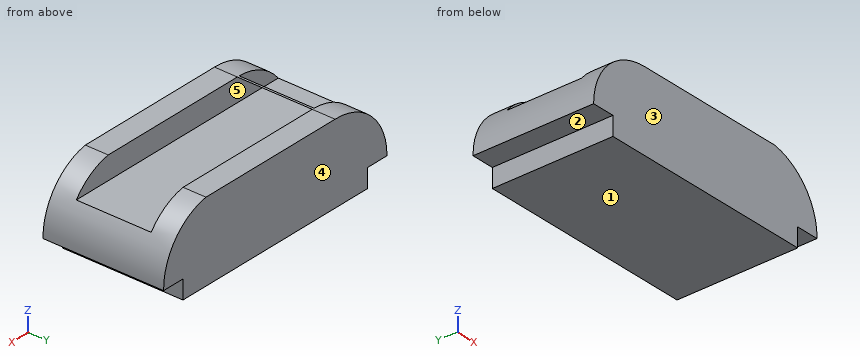
from build123d import *

# Parameters (mm, degrees)
F1_DEPTH      = 29
F2_W          = 36
F2_H          = 11
F3_DEPTH      = 66.5054850399
F3_DEPTH_BACK = 60.4995857167


with BuildPart() as f1:
    # F0 (on Front) → F1 (new body, symmetric)
    with BuildSketch(Plane.XZ):
        with BuildLine():
            Line((-55.504484674, 9), (-55.504484674, 0))
            Line((-55.504484674, 0), (49.495515326, 0))
            Line((49.495515326, 0), (49.495515326, 9))
            Line((49.495515326, 9), (60.495515326, 9))
            ThreePointArc((60.495515326, 9), (53.8144067162, 27.9423579991), (36.4278033617, 38))
            Line((36.4278033617, 38), (-36.987580359, 38))
            ThreePointArc((-36.987580359, 38), (-57.8286498328, 29.6910356314), (-66.504484674, 9))
            Line((-66.504484674, 9), (-55.504484674, 9))
        make_face()
    extrude(amount=F1_DEPTH, both=True)

    # F2 (on Right) → F3 (cut, two sides)
    with BuildSketch(Plane.YZ) as f3_sk:
        with Locations((0, 32.5)):
            Rectangle(F2_W, F2_H)
    extrude(amount=-F3_DEPTH, mode=Mode.SUBTRACT)
    extrude(f3_sk.sketch, amount=F3_DEPTH_BACK, mode=Mode.SUBTRACT)


solid = f1.part
Check sheet for the modelled part. Datum: model origin and axes. Units: mm. Face numbers are marked on the shaded views. A direction names the side the tool comes from. Coordinates: 2 decimals unless noted, no trailing zeros. Loops run counter-clockwise (first coordinate to the right, second up) from the corner with the lowest first, then second, coordinate; pieces in that order, holes last. Notation, with made-up numbers: (-14.5, -28) -> (32.5, -28) arc R21 cw to (32.5, -8) -> close; hole circle Ø10 at (-33.75, -23). An arc over 180 degrees is marked (long way). Write item = value, one per line. Start each with the question number.
1. Draft check along Y on the marked faces 3, 4 and 5. Enter one of: released by +Y, released by -Y, zero draft, split by the parting line, or undercut.
2. Material ranges on line 1 (Y direction, x = -27.5, z = 32); line 2 (Z direction, x = -13, y = -16); line 3 (X direction, y = 5, z = 7), recorded low to high.
3. Section check D-D on z = 3. Record the cut outline in (x, y), then the cut area to 3 significant figures.
4. Section check B-B on z = 36.5. Record the cut outline in (x, y), then the cut area to 3 significant figures.
5. Depth check by flat-ended pin: P1, Ø5.5, axis at x = -2.5, y = 24, coming from the +Z side; P2, Ø7, axis at y = -12, z = 2.5, coming from the +X side; P3, Ø12, axis at y = -21, z = 23, coming from the -X side. Enter the tip coordinate at first touch or a pass-through.
6. Section check C-C on x = -17. Record the cut outline in (y, z).
7. Tool access check on the marked faces 1 and 2. Record the directions out of +Z, -Z, +X, -X, +Y, -Y that give a thin tool (end or side, any length) a straight path to the whole face; none if there is none.
Responses:
q1.face_3 = released by -Y
q1.face_4 = released by +Y
q1.face_5 = undercut
q2.line_1 = -29 to -18, 18 to 29
q2.line_2 = 0 to 27
q2.line_3 = -55.5 to 49.5
q3.outline = (-55.5, -29) -> (49.5, -29) -> (49.5, 29) -> (-55.5, 29) -> close
q3.area = 6,090 mm2
q4.outline = (-46.72, -29) -> (41.88, -29) -> (41.88, -18) -> (-46.72, -18) -> close; (-46.72, 18) -> (41.88, 18) -> (41.88, 29) -> (-46.72, 29) -> close
q4.area = 1,950 mm2
q5.P1 = 38
q5.P2 = 49.5
q5.P3 = -65.38
q6.outline = (-29, 0) -> (29, 0) -> (29, 38) -> (18, 38) -> (18, 27) -> (-18, 27) -> (-18, 38) -> (-29, 38) -> close
q7.face_1 = -Z, +X, -X, +Y, -Y
q7.face_2 = -Z, -X, +Y, -Y
